Geometry check sheet. Reference: the model listing, model coordinates, mm. Face numbers are marked on the shaded views. Round coordinates to 2 decimals unless told otherwise and drop trailing zeros. Loops run counter-clockwise (first coordinate to the right, second up) from the corner with the lowest first, then second, coordinate; pieces in that order, holes last. Notation, with made-up numbers: (84.5, 79) -> (123.5, 79) arc R31 cw to (123.5, 112) -> close; hole circle Ø6 at (47.25, -28.5). An arc over 180 degrees is marked (long way). Use a Markdown table: item, result. Add a question column.
Q1. Sectioned sample at B-B, the plane z = 6.35. Give the number of separate pieces and of enclosed holes in the cut face, then the cut area to 3 significant figures.
Q2. Sectioned sample at A-A, the plane x = 0. Enter the section's corners in (y, z) (3 decimals).
Q3. Release check for a two-part mould opening along Y. For the marked faces 1, 2, 3 and 4 record: released by +Y, released by -Y, zero draft, split by the parting line, or undercut.
Q4. Material ranges on L1, parallel to Y at x = 2.5, z = 6.35 (3 decimals); L2, parallel to Y at x = 1.5, z = 6.35 (3 decimals); L3, parallel to Y at x = 1.75, z = 6.35 (3 decimals), recorded low to high.
Q5. Sectioned sample at C-C, the plane y = -1.5. Enter the section's corners in (x, z), then the cut area to 3 significant figures.
Q6. Gauge pin test, flat end, axial feed: P1, Ø2.5, axis at x = 0, y = -3.175, coming from the -Z side. Record the tip position at first contact, or that the pin passes through.
Autodesk Inventor part; units mm, degrees
ref_plane "YZ Plane" through (0, 0, 0) normal (1, 0, 0) x (0, 1, 0)
ref_plane "XZ Plane" through (0, 0, 0) normal (0, 1, 0) x (-1, 0, 0)
ref_plane "XY Plane" through (0, 0, 0) normal (0, 0, 1) x (1, 0, 0)
sketch "Sketch1" plane through (0, 0, 0) normal (0, 0, 1) x (1, 0, 0)
  line L0 (-6.35, -9.525) -> (6.35, -9.525)
  line L1 (6.35, -9.525) -> (6.35, 9.525)
  line L2 (6.35, 9.525) -> (-6.35, 9.525)
  line L3 (-6.35, 9.525) -> (-6.35, -9.525)
  line L4 (-6.35, -9.525) -> (6.35, 9.525) construction
  line L5 (6.35, -9.525) -> (-6.35, 9.525) construction
  point P0 (0, 0)
  dimension "d0" = 12.7
  dimension "d1" = 19.05
extrude "Plate1" add sketch "Sketch1" along normal blind 12.7
sketch "Sketch2" plane through (6.35, -9.525, 0) normal (1, 0, 0) x (0, 0, -1)
  line L0 (0, 19.05) -> (-12.7, 19.05)
  line L1 (0, 0) -> (0, 19.05)
  point P0 (0, 9.525)
  point P1 (-6.35, 12.7)
  dimension "d3" = 6.35
  dimension "d4" = 6.35
hole "Hole1" at (6.35, 3.175, 6.35) direction (-1, 0, 0) diameter 3.9624 depth 12.7 tip angle 118
sketch "Sketch3" plane through (0, 0, 12.7) normal (0, 0, 1) x (1, 0, 0)
  line L0 (6.35, -9.525) -> (-6.35, -9.525)
  point P0 (0, 0)
  point P1 (0, -3.175)
  dimension "d12" = 6.35
hole "Hole2" at (0, -3.175, 12.7) direction (0, 0, -1) diameter 3.9624 depth 12.7 tip angle 118
fillet "Corner Round1" radius 1.5875 4 edges at (6.35, -9.525, 6.35) (-6.35, 9.525, 6.35) (6.35, 9.525, 6.35) (-6.35, -9.525, 6.35)
equation "\"d10\" = Thickness"
equation "\"d18\" = Thickness"
equation "\"d2\" = Thickness"
equation "\"BendRadius\" = Thickness"
equation "\"BendReliefWidth\" = Thickness"
equation "\"BendReliefDepth\" = 0.5 * Thickness"
equation "\"CornerReliefSize\" = 4 * Thickness"
equation "\"MinimumRemnant\" = 2 * Thickness"
equation "\"TransitionRadius\" = BendRadius"
equation "\"JacobiRadiusSize\" = BendRadius"
equation "\"GapSize\" = Thickness"
properties part number "PLATE,NUT-BLOCK,1-LONG" material "Aluminum 6061"
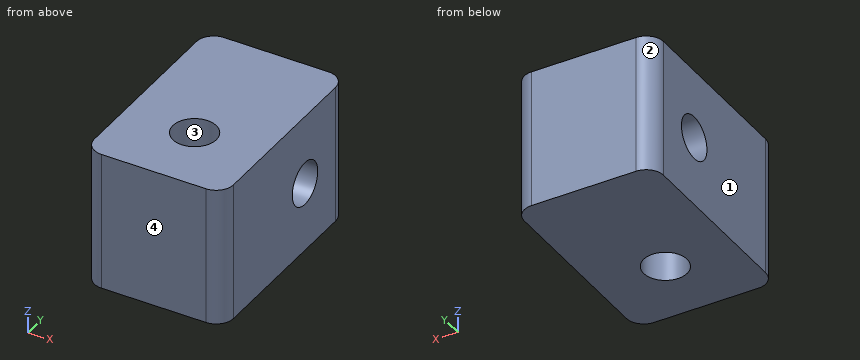
Values:
| question | item | result |
|---|---|---|
| 1 | separate pieces | 2 |
| 1 | enclosed holes | 1 |
| 1 | area | 177 mm^2 |
| 2 | outline | (-9.525, 0) -> (-5.156, 0) -> (-5.156, 12.7) -> (-9.525, 12.7) -> close; (-1.194, 0) -> (9.525, 0) -> (9.525, 12.7) -> (-1.194, 12.7) -> close; hole circle Ø3.962 at (3.175, 6.35) |
| 3 | face 1 | zero draft |
| 3 | face 2 | released by +Y |
| 3 | face 3 | undercut |
| 3 | face 4 | released by -Y |
| 4 | L1 | -9.525 to 1.194, 5.156 to 9.525 |
| 4 | L2 | -9.525 to -4.469, -1.881 to 1.194, 5.156 to 9.525 |
| 4 | L3 | -9.525 to -4.104, -2.246 to 1.194, 5.156 to 9.525 |
| 5 | outline | (-6.35, 0) -> (-1.06, 0) -> (-1.06, 12.7) -> (-6.35, 12.7) -> close; (1.06, 0) -> (6.35, 0) -> (6.35, 12.7) -> (1.06, 12.7) -> close |
| 5 | area | 134 mm^2 |
| 6 | P1 | through |
